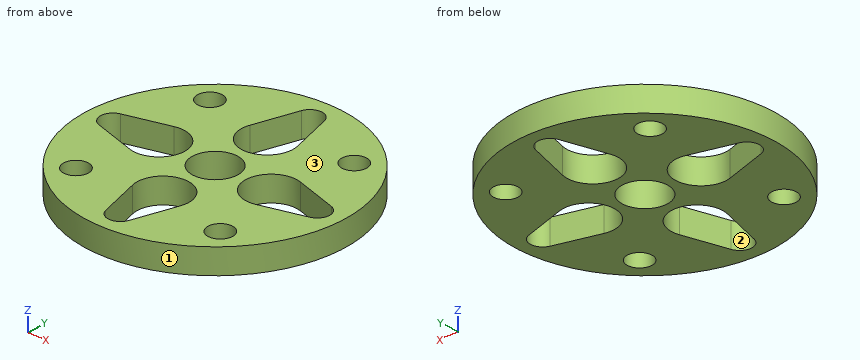
```python
from build123d import *

# Parameters (mm, degrees)
MODEL_R                 = 15.73
MODEL_R_2               = 1.5
MODEL_R_3               = 2.75
SALIENTE_EXTRUIR1_DEPTH = 3


with BuildPart() as part:
    # Model → Saliente-Extruir1 (new body)
    with BuildSketch(Plane.XY):
        with Locations((22.468172618, 284.73044756)):
            Circle(MODEL_R)
        with Locations((13.468172618, 275.73044756)):
            Circle(MODEL_R_2, mode=Mode.SUBTRACT)
        with Locations((31.468172618, 275.73044756)):
            Circle(MODEL_R_2, mode=Mode.SUBTRACT)
        with Locations((31.468172618, 293.73044756)):
            Circle(MODEL_R_2, mode=Mode.SUBTRACT)
        with Locations((13.468172618, 293.73044756)):
            Circle(MODEL_R_2, mode=Mode.SUBTRACT)
        with Locations((22.468172618, 284.73044756)):
            Circle(MODEL_R_3, mode=Mode.SUBTRACT)
        with BuildLine():
            Line((23.908463874, 297.877369736), (25.444774548, 292.59638113))
            ThreePointArc((25.444774548, 292.59638113), (22.468172618, 288.63044756), (19.491570687, 292.59638113))
            Line((19.491570687, 292.59638113), (21.027881361, 297.877369736))
            ThreePointArc((21.027881361, 297.877369736), (22.468172618, 298.958369621), (23.908463874, 297.877369736))
        make_face(mode=Mode.SUBTRACT)
        with BuildLine():
            Line((9.321250442, 286.170738816), (14.602239048, 287.70704949))
            ThreePointArc((14.602239048, 287.70704949), (18.568172618, 284.73044756), (14.602239048, 281.753845629))
            Line((14.602239048, 281.753845629), (9.321250442, 283.290156303))
            ThreePointArc((9.321250442, 283.290156303), (8.240250556, 284.73044756), (9.321250442, 286.170738816))
        make_face(mode=Mode.SUBTRACT)
        with BuildLine():
            Line((21.027881361, 271.583525384), (19.491570687, 276.86451399))
            ThreePointArc((19.491570687, 276.86451399), (22.468172618, 280.83044756), (25.444774548, 276.86451399))
            Line((25.444774548, 276.86451399), (23.908463874, 271.583525384))
            ThreePointArc((23.908463874, 271.583525384), (22.468172618, 270.502525498), (21.027881361, 271.583525384))
        make_face(mode=Mode.SUBTRACT)
        with BuildLine():
            Line((35.615094794, 283.290156303), (30.334106188, 281.753845629))
            ThreePointArc((30.334106188, 281.753845629), (26.368172618, 284.73044756), (30.334106188, 287.70704949))
            Line((30.334106188, 287.70704949), (35.615094794, 286.170738816))
            ThreePointArc((35.615094794, 286.170738816), (36.696094679, 284.73044756), (35.615094794, 283.290156303))
        make_face(mode=Mode.SUBTRACT)
    extrude(amount=SALIENTE_EXTRUIR1_DEPTH)


solid = part.part
```
Design review of the part built by this model. Coordinates are the model's own, in mm. Face numbers are marked on the shaded views. Round coordinates to 2 decimals unless told otherwise and drop trailing zeros. Order: outer loops, then holes, each group sorted by start corner. A loop starts at its lowest first (then second) coordinate and runs counter-clockwise, first axis right, second up. Notation, with made-up numbers: (61.5, 86) - (71.5, 86) arc R24 ccw to (71.5, 106) - close; hole circle Ø9 at (-26.5, 79.5). An arc over 180 degrees is marked (long way). One line per question, with ' | ' between items.
Item 1: Take a section at A-A, the plane y = 296.5. Write out the cut boundary in (x, z), then the cut area to 3 significant figures.
Checks:
outline: (12.03, 0) - (20.63, 0) - (20.63, 3) - (12.03, 3) - close; (24.31, 0) - (32.9, 0) - (32.9, 3) - (24.31, 3) - close | area: 51.6 mm²
Item 2: Draft analysis for pull direction Y (two halves, no side actions). For the marked faces 1, 2 and 3, state which applies: +Y half, -Y half, draft (parallel to the pull), parting line (faces both ways), or undercut.
Checks:
face 1: parting line | face 2: undercut | face 3: draft
Item 3: Take a section at C-C, the plane z = 1.65. Give the number of separate pieces and of enclosed holes in the cut face, then the cut area to 3 significant figures.
Checks:
separate pieces: 1 | enclosed holes: 9 | area: 541 mm²
Item 4: For P1, Ø1, axis at x = 14, z = 1.5, coming from the -Y side; P2, Ø3.5, axis at x = 13.47, y = 275.73, coming from the -Z side; P3, Ø1, axis at x = 35, z = 2, coming from the -Y side, all flat-tipped, find the tip position at first contact; note any pin that passes through.
Checks:
P1: y = 271.17 | P2: z = 0 | P3: y = 274.6
Item 5: Take a section at D-D, the plane y = 275. Write out the cut boundary in (x, z).
Checks:
outline: (10.11, 0) - (12.16, 0) - (12.16, 3) - (10.11, 3) - close; (14.78, 0) - (20.03, 0) - (20.03, 3) - (14.78, 3) - close; (24.9, 0) - (30.16, 0) - (30.16, 3) - (24.9, 3) - close; (32.78, 0) - (34.83, 0) - (34.83, 3) - (32.78, 3) - close
Item 6: Wall thickness on line 1 (X direction, y = 286, z = 2.1) (3 decimals); line 2 (X direction, y = 275, z = 1.45); line 3 (Y direction, x = 36, z = 1.3): over which ranges is each line inside the solid? List them lowest first. Write a range as [from, to].
Checks:
line 1: [6.789, 8.941], [18.296, 20.029], [24.908, 26.64], [35.995, 38.147] | line 2: [10.11, 12.16], [14.78, 20.03], [24.9, 30.16], [32.78, 34.83] | line 3: [276.71, 283.46], [286, 292.75]
Item 7: Take a section at B-B, the plane x = 34. Write out the cut boundary in (y, z).
Checks:
outline: (274.03, 0) - (282.82, 0) - (282.82, 3) - (274.03, 3) - close; (286.64, 0) - (295.43, 0) - (295.43, 3) - (286.64, 3) - close
